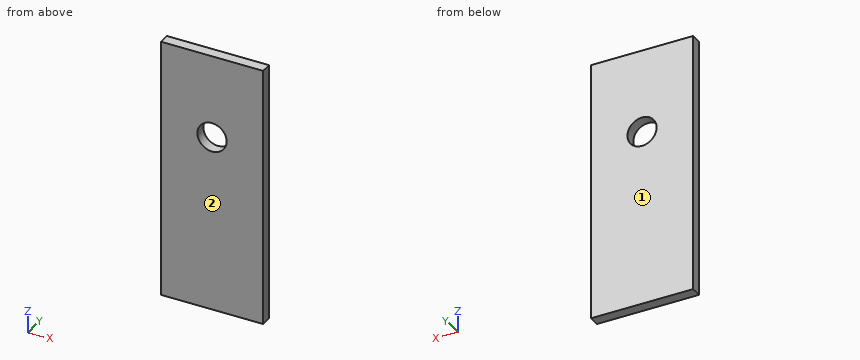
from build123d import *

# Parameters (mm, degrees)
SKETCH1_W           = 28
SKETCH1_H           = 71.2
BOSS_EXTRUDE1_DEPTH = 3
SKETCH4_R           = 1
CUT_EXTRUDE2_DEPTH  = 10
SKETCH5_R           = 4
CUT_EXTRUDE3_DEPTH  = 10
SKETCH10_R          = 1.75
CUT_EXTRUDE9_DEPTH  = 1.6
SKETCH12_R          = 1.75
BOSS_EXTRUDE2_DEPTH = 3


with BuildPart() as part:
    # Sketch1 → Boss-Extrude1 (new body)
    with BuildSketch(Plane(origin=(0, 0, 0), x_dir=(1, 0, 0), z_dir=(0, 1, 0))):
        Rectangle(SKETCH1_W, SKETCH1_H)
    extrude(amount=BOSS_EXTRUDE1_DEPTH)

    # Sketch4 → Cut-Extrude2 (cut)
    with BuildSketch(Plane(origin=(0, 3, 0), x_dir=(1, 0, 0), z_dir=(0, 1, 0))):
        with Locations((7, -12.8)):
            Circle(SKETCH4_R)
        with Locations((0, -19.8)):
            Circle(SKETCH4_R)
        with Locations((-7, -12.8)):
            Circle(SKETCH4_R)
        with Locations((0, -5.8)):
            Circle(SKETCH4_R)
    extrude(amount=-CUT_EXTRUDE2_DEPTH, mode=Mode.SUBTRACT)

    # Sketch5 → Cut-Extrude3 (cut)
    with BuildSketch(Plane(origin=(0, 3, 0), x_dir=(1, 0, 0), z_dir=(0, 1, 0))):
        with Locations((0, -12.8)):
            Circle(SKETCH5_R)
    extrude(amount=-CUT_EXTRUDE3_DEPTH, mode=Mode.SUBTRACT)

    # Sketch10 → Cut-Extrude9 (cut)
    with BuildSketch(Plane(origin=(0, 3, 0), x_dir=(1, 0, 0), z_dir=(0, 1, 0))):
        with Locations((0, -19.8)):
            Circle(SKETCH10_R)
        with Locations((-7, -12.8)):
            Circle(SKETCH10_R)
        with Locations((0, -5.8)):
            Circle(SKETCH10_R)
        with Locations((7, -12.8)):
            Circle(SKETCH10_R)
    extrude(amount=-CUT_EXTRUDE9_DEPTH, mode=Mode.SUBTRACT)

    # Sketch12 → Boss-Extrude2 (add)
    with BuildSketch(Plane(origin=(0, 3, 0), x_dir=(1, 0, 0), z_dir=(0, 1, 0))):
        with Locations((0, -19.8)):
            Circle(SKETCH12_R)
        with Locations((-7, -12.8)):
            Circle(SKETCH12_R)
        with Locations((0, -5.8)):
            Circle(SKETCH12_R)
        with Locations((7, -12.8)):
            Circle(SKETCH12_R)
    extrude(amount=-BOSS_EXTRUDE2_DEPTH)


solid = part.part
The listing builds one solid part. Answer for the finished solid, in the listing's coordinates (mm). Face numbers are marked on the shaded views. Give positions to 0.01 mm unless a question says otherwise; leave off trailing zeros. Write each loop counter-clockwise with the first axis right and the second up, starting at its lowest first coordinate (ties: lowest second). Pieces come first, ordered by that corner, then holes.
Item 1: Section C-C, the plane y = 2.3 is taken. Write down the section's boundary in (x, z), plus the area to 3 significant figures.
Item 2: Find the intervals of material crossed by line 1 along X through (y, z) = (0.8, 12.8); line 2 along Z through (x, y) = (0, 1.8); line 3 along Z through (x, y) = (-2.75, 2.75), in increasing order.
Item 3: Section A-A, the plane z = 12.8 is taken. Write down the section's boundary in (x, y).
Item 4: Determine the mould class of the marked faces 1 and 2 for opening direction Y: released by +Y, released by -Y, zero draft, split by the parting line, or undercut.
Item 5: Section B-B, the plane x = 1.75 is taken. Write down the section's boundary in (y, z), plus the area to 3 significant figures.
Completed:
1. outline: (-14, -35.6) - (14, -35.6) - (14, 35.6) - (-14, 35.6) - close; hole circle Ø8 at (0, 12.8)
1. area: 1,940 mm2
2. line 1: x = -14 to -4, 4 to 14
2. line 2: z = -35.6 to 8.8, 16.8 to 35.6
2. line 3: z = -35.6 to 9.9, 15.7 to 35.6
3. outline: (-14, 0) - (-4, 0) - (-4, 3) - (-14, 3) - close; (4, 0) - (14, 0) - (14, 3) - (4, 3) - close
4. face 1: released by +Y
4. face 2: released by -Y
5. outline: (0, -35.6) - (3, -35.6) - (3, 9.2) - (0, 9.2) - close; (0, 16.4) - (3, 16.4) - (3, 35.6) - (0, 35.6) - close
5. area: 192 mm2
